The model under review builds one solid part; all positions refer to its coordinate system, in mm. A direction names the side the tool comes from. Coordinates: 2 decimals unless noted, no trailing zeros. Order: outer loops, then holes, each group sorted by start corner. A loop starts at its lowest first (then second) coordinate and runs counter-clockwise, first axis right, second up. Notation, with made-up numbers: M 11.25,-17.75 L 47.25,-17.75 A35 ccw 47.25,19.25 Z; hole C 35.5,13.5 d3. An arc over 180 degrees is marked long. One line per item, written item: value.
Autodesk Inventor part; units mm, degrees
ref_plane "YZ Plane" through (0, 0, 0) normal (1, 0, 0) x (0, 1, 0)
ref_plane "XZ Plane" through (0, 0, 0) normal (0, 1, 0) x (-1, 0, 0)
ref_plane "XY Plane" through (0, 0, 0) normal (0, 0, 1) x (1, 0, 0)
sketch "Boceto1" plane through (0, 0, 0) normal (0, 1, 0) x (-1, 0, 0)
  line L0 (0, 0) -> (-93, 0)
  line L1 (-93, 0) -> (-93, -118)
  line L2 (-93, -118) -> (0, -118)
  line L3 (0, -118) -> (0, 0)
  dimension "d0" = 93
  dimension "d1" = 118
extrude "Extrusión1" add sketch "Boceto1" along normal blind 6
shell "Vaciado1" thickness 3 removed faces 1 at (62, 6, -39.3333)
sketch "Boceto11" plane through (3, 3, -3) normal (0, 1, 0) x (1, 0, 0)
  line L0 (40, 70) -> (45, 70)
  line L1 (45, 70) -> (45, 63)
  line L2 (45, 63) -> (40, 63)
  line L3 (40, 63) -> (40, 70)
  line L4 (40, 48) -> (45, 48)
  line L5 (45, 48) -> (45, 41)
  line L6 (45, 41) -> (40, 41)
  line L7 (40, 41) -> (40, 48)
  point P0 (-3, -3)
  dimension "d33" = 5
  dimension "d34" = 7
  dimension "d35" = 5
  dimension "d36" = 7
extrude "Extrusión8" cut sketch "Boceto11" against normal blind 7
sketch "Boceto12" plane through (0, 0, 0) normal (0, -1, 0) x (1, 0, 0)
  line L0 (28, -28) -> (38, -28)
  line L1 (38, -28) -> (38, -38)
  line L2 (38, -38) -> (28, -38)
  line L3 (28, -38) -> (28, -28)
  line L4 (55, -38) -> (65, -38)
  line L5 (65, -38) -> (65, -28)
  line L6 (65, -28) -> (55, -28)
  line L7 (55, -28) -> (55, -38)
  point P0 (0, 0)
  dimension "d39" = 10
  dimension "d40" = 10
  dimension "d41" = 10
  dimension "d42" = 10
extrude "Extrusión9" add sketch "Boceto12" along normal blind 40
sketch "Boceto13" plane through (28, 0, -38) normal (-1, 0, 0) x (0, 0, 1)
  line L0 (10, -40) -> (0, -40)
  line L1 (0, -40) -> (10, -35.9597)
  line L2 (10, 0) -> (10, -40)
  line L3 (0, -40) -> (10.7853, -40) construction
  point P0 (38, 0)
  dimension "d45" = 22
extrude "Extrusión10" cut sketch "Boceto13" against normal blind 40
sketch "Boceto14" plane through (28, -35.9597, -28) normal (0, -0.9272, 0.3746) x (1, 0, 0)
  line L0 (0, 13.4708) -> (0, 0)
  line L1 (0, 0) -> (-10, 0)
  line L2 (-10, 0) -> (-10, -10)
  line L3 (-10, -10) -> (0, -10)
  line L4 (0, -10) -> (0, 0)
  line L5 (37, 0) -> (37, -10.7853)
  line L6 (37, -10.7853) -> (47, -10.7853)
  line L7 (47, -10.7853) -> (47, -0.7853)
  line L8 (47, -0.7853) -> (37, -0.7853)
  line L9 (37, -0.7853) -> (37, -10.7853)
  point P0 (-28, 39.4319)
  point P1 (37, -0.7853)
  dimension "d48" = 10
  dimension "d49" = 10
  dimension "d50" = 10
  dimension "d51" = 10
extrude "Extrusión11" add sketch "Boceto14" against normal blind 10
fillet "Empalme1" radius 2 12 edges at (93, 6, -59) (93, 0, -59) (46.5, 0, -118) (46.5, 6, -118) (0, 6, -59) (0, 0, -59) (0, 3, -118) (93, 3, -118) (0, 3, 0) (46.5, 6, 0) (46.5, 0, 0) (93, 3, 0)
properties part number "Piezatapa"
(1) Tool access review of faces 1 (the flat face through (22.93, -35.13, -39.12)), 2 (the flat face through (3, 4, -60)), 3 (the flat face through (65, -33, -40)), 4 (the flat face through (18, -33, -34)): name each direction out of +Z, -Z, +X, -X, +Y, -Y from which nothing blocks a thin tool from reaching the whole face with its end or side.
Geometry results:
face 1: -Z, -X, -Y
face 2: +Y
face 3: -Z, -Y
face 4: +Z, -Z, -X, -Y
(2) We need section D-D, the plane x = 80.5. State the section outline as (y, z) points.
Geometry results:
outline: M 0,-116 A2 ccw 2,-118 L 4,-118 A2 ccw 6,-116 L 6,-115 L 3,-115 L 3,-3 L 6,-3 L 6,-2 A2 ccw 4,0 L 2,0 A2 ccw 0,-2 Z
(3) Insertion check: pin 1 Ø10 at (y, z) = (-27.5, -25) entering from -X; pin 2 Ø1 at (x, y) = (30, -25) entering from +Z; pin 3 Ø1.9 at (y, z) = (-35, -40) entering from -X. Each pin has a flat end and moves straight along its axis. Give the tip position at first contact, or say it passes through.
Geometry results:
pin 1: stops at x = 28
pin 2: stops at z = -28
pin 3: stops at x = 18
(4) We need section A-A, the plane y = -16.5. State the section outline as (x, z) points, plus the area to 3 significant figures.
Geometry results:
outline: M 28,-38 L 38,-38 L 38,-28 L 28,-28 Z; M 55,-38 L 65,-38 L 65,-28 L 55,-28 Z
area: 200 mm2
(5) Mouldability with a two-part tool opening along Z and no side actions: class faces 5 (the flat face through (23.07, -31.389, -29.847)), 6 (the flat face through (75, -34, -35)), 7 (the flat face through (46, 4, -3)), 8 (the flat face through (69.93, -35.429, -39.847)) as +Z half, -Z half, draft (parallel to the pull), parting line (faces both ways), or undercut.
Geometry results:
face 5: +Z half
face 6: draft
face 7: undercut
face 8: -Z half
(6) We need section C-C, the plane z = -46. State the section outline as (x, y) points, plus the area to 3 significant figures.
Geometry results:
outline: M 0,2 A2 ccw 2,0 L 43,0 L 43,3 L 3,3 L 3,6 L 2,6 A2 ccw 0,4 Z; M 48,0 L 91,0 A2 ccw 93,2 L 93,4 A2 ccw 91,6 L 90,6 L 90,3 L 48,3 Z
area: 279 mm2
(7) We need section B-B, the plane x = 66.5. State the section outline as (y, z) points.
Geometry results:
outline: M -40,-38 L -30.73,-41.75 L -26.98,-32.47 L -36.25,-28.73 Z; M 0,-116 A2 ccw 2,-118 L 4,-118 A2 ccw 6,-116 L 6,-115 L 3,-115 L 3,-3 L 6,-3 L 6,-2 A2 ccw 4,0 L 2,0 A2 ccw 0,-2 Z
(8) For L1, parallel to X at y = 4, z = -47.5; L2, parallel to X at y = -14, z = -29; L3, parallel to Y at x = 71.5, z = -45.5, list the stretches that pass through material, from the lowest coordinate up.
Geometry results:
L1: x = 0 to 3, 90 to 93
L2: x = 28 to 38, 55 to 65
L3: y = 0 to 3
